Geometry check sheet. Reference: the model listing, model coordinates, mm. A direction names the side the tool comes from. Coordinates: 2 decimals unless noted, no trailing zeros. Write each loop counter-clockwise with the first axis right and the second up, starting at its lowest first coordinate (ties: lowest second). Pieces come first, ordered by that corner, then holes. Notation, with made-up numbers: M 35,66.5 L 92,66.5 A17 ccw 92,89.5 Z; hole C 66.25,75.25 d1. An arc over 180 degrees is marked long. Write item = value, one per line. Start each with the question number.
```python
from build123d import *

# Parameters (mm, degrees)
BOX017_W      = 3
BOX017_H      = 3
BOX017_DEPTH  = 3
BOX018_W      = 3
BOX018_H      = 3
BOX018_DEPTH  = 3
BOX019_W      = 3
BOX019_H      = 3
BOX019_DEPTH  = 3
BOX016_W      = 3
BOX016_H      = 3
BOX016_DEPTH  = 3
BOX012_W      = 3.1
BOX012_H      = 6
BOX012_DEPTH  = 10
BOX013_W      = 3.1
BOX013_H      = 6
BOX013_DEPTH  = 10
BOX014_W      = 6
BOX014_H      = 3.1
BOX014_DEPTH  = 10
BOX015_W      = 6
BOX015_H      = 3.1
BOX015_DEPTH  = 10
BOX001_W      = 3.1
BOX001_H      = 6
BOX001_DEPTH  = 3
BOX002_W      = 6
BOX002_H      = 3.1
BOX002_DEPTH  = 3
BOX003_W      = 6
BOX003_H      = 3.1
BOX003_DEPTH  = 3
BOX_W         = 3.1
BOX_H         = 6
BOX_DEPTH     = 3
TUBE001_R     = 16.7
TUBE001_R_2   = 15.7
TUBE001_DEPTH = 10
BOX005_W      = 1
BOX005_H      = 16
BOX005_DEPTH  = 10
BOX006_W      = 1
BOX006_H      = 16
BOX006_DEPTH  = 10
BOX007_W      = 1
BOX007_H      = 16
BOX007_DEPTH  = 10
BOX008_W      = 16
BOX008_H      = 1
BOX008_DEPTH  = 10
BOX009_W      = 16
BOX009_H      = 1
BOX009_DEPTH  = 10
BOX010_W      = 16
BOX010_H      = 1
BOX010_DEPTH  = 10
BOX011_W      = 16
BOX011_H      = 1
BOX011_DEPTH  = 10
BOX004_W      = 1
BOX004_H      = 16
BOX004_DEPTH  = 10
TUBE_R        = 32.5
TUBE_R_2      = 15.7
TUBE_DEPTH    = 3


with BuildPart() as finlock002:
    # Box017 → Box017 (new body)
    with BuildSketch(Plane(origin=(-1.5, 21, -3), x_dir=(1, 0, 0), z_dir=(0, 0, 1))):
        with Locations((1.5, 1.5)):
            Rectangle(BOX017_W, BOX017_H)
    extrude(amount=BOX017_DEPTH)


with BuildPart() as finlock003:
    # Box018 → Box018 (new body)
    with BuildSketch(Plane(origin=(-1.5, -24, -3), x_dir=(1, 0, 0), z_dir=(0, 0, 1))):
        with Locations((1.5, 1.5)):
            Rectangle(BOX018_W, BOX018_H)
    extrude(amount=BOX018_DEPTH)


with BuildPart() as finlock004:
    # Box019 → Box019 (new body)
    with BuildSketch(Plane(origin=(-24, -1.5, -3), x_dir=(1, 0, 0), z_dir=(0, 0, 1))):
        with Locations((1.5, 1.5)):
            Rectangle(BOX019_W, BOX019_H)
    extrude(amount=BOX019_DEPTH)


with BuildPart() as finlocks:
    # Box016 → Box016 (new body)
    with BuildSketch(Plane(origin=(21, -1.5, -3), x_dir=(1, 0, 0), z_dir=(0, 0, 1))):
        with Locations((1.5, 1.5)):
            Rectangle(BOX016_W, BOX016_H)
    extrude(amount=BOX016_DEPTH)

    # Fusion005: union FinLock002, FinLock003, FinLock004
    add(finlock002.part)
    add(finlock003.part)
    add(finlock004.part)


with BuildPart() as fincut005:
    # Box012 → Box012 (new body)
    with BuildSketch(Plane(origin=(-1.55, -21, -10), x_dir=(1, 0, 0), z_dir=(0, 0, 1))):
        with Locations((1.55, 3)):
            Rectangle(BOX012_W, BOX012_H)
    extrude(amount=BOX012_DEPTH)


with BuildPart() as fincut006:
    # Box013 → Box013 (new body)
    with BuildSketch(Plane(origin=(-1.55, 15, -10), x_dir=(1, 0, 0), z_dir=(0, 0, 1))):
        with Locations((1.55, 3)):
            Rectangle(BOX013_W, BOX013_H)
    extrude(amount=BOX013_DEPTH)


with BuildPart() as fincut007:
    # Box014 → Box014 (new body)
    with BuildSketch(Plane(origin=(15, -1.55, -10), x_dir=(1, 0, 0), z_dir=(0, 0, 1))):
        with Locations((3, 1.55)):
            Rectangle(BOX014_W, BOX014_H)
    extrude(amount=BOX014_DEPTH)


with BuildPart() as innerfincutouts:
    # Box015 → Box015 (new body)
    with BuildSketch(Plane(origin=(-21, -1.55, -10), x_dir=(1, 0, 0), z_dir=(0, 0, 1))):
        with Locations((3, 1.55)):
            Rectangle(BOX015_W, BOX015_H)
    extrude(amount=BOX015_DEPTH)

    # Fusion002: union FinCut005, FinCut006, FinCut007
    add(fincut005.part)
    add(fincut006.part)
    add(fincut007.part)


with BuildPart() as fincut002:
    # Box001 → Box001 (new body)
    with BuildSketch(Plane(origin=(-1.55, 28, 0), x_dir=(1, 0, 0), z_dir=(0, 0, 1))):
        with Locations((1.55, 3)):
            Rectangle(BOX001_W, BOX001_H)
    extrude(amount=BOX001_DEPTH)


with BuildPart() as fincut003:
    # Box002 → Box002 (new body)
    with BuildSketch(Plane(origin=(28, -1.55, 0), x_dir=(1, 0, 0), z_dir=(0, 0, 1))):
        with Locations((3, 1.55)):
            Rectangle(BOX002_W, BOX002_H)
    extrude(amount=BOX002_DEPTH)


with BuildPart() as fincut004:
    # Box003 → Box003 (new body)
    with BuildSketch(Plane(origin=(-34, -1.55, 0), x_dir=(1, 0, 0), z_dir=(0, 0, 1))):
        with Locations((3, 1.55)):
            Rectangle(BOX003_W, BOX003_H)
    extrude(amount=BOX003_DEPTH)


with BuildPart() as fincutouts:
    # Box → Box (new body)
    with BuildSketch(Plane(origin=(-1.55, -34, 0), x_dir=(1, 0, 0), z_dir=(0, 0, 1))):
        with Locations((1.55, 3)):
            Rectangle(BOX_W, BOX_H)
    extrude(amount=BOX_DEPTH)

    # Fusion: union FinCut002, FinCut003, FinCut004
    add(fincut002.part)
    add(fincut003.part)
    add(fincut004.part)

    # Fusion003: union InnerFinCutouts
    add(innerfincutouts.part)


with BuildPart() as innertube:
    # Tube001 → Tube001 (new body)
    with BuildSketch(Plane.XY.offset(-10)):
        Circle(TUBE001_R)
        Circle(TUBE001_R_2, mode=Mode.SUBTRACT)
    extrude(amount=TUBE001_DEPTH)


with BuildPart() as alignment002:
    # Box005 → Box005 (new body)
    with BuildSketch(Plane(origin=(-2.7, 16, -10), x_dir=(1, 0, 0), z_dir=(0, 0, 1))):
        with Locations((0.5, 8)):
            Rectangle(BOX005_W, BOX005_H)
    extrude(amount=BOX005_DEPTH)


with BuildPart() as alignment003:
    # Box006 → Box006 (new body)
    with BuildSketch(Plane(origin=(-2.7, -32, -10), x_dir=(1, 0, 0), z_dir=(0, 0, 1))):
        with Locations((0.5, 8)):
            Rectangle(BOX006_W, BOX006_H)
    extrude(amount=BOX006_DEPTH)


with BuildPart() as alignment004:
    # Box007 → Box007 (new body)
    with BuildSketch(Plane(origin=(1.7, -32, -10), x_dir=(1, 0, 0), z_dir=(0, 0, 1))):
        with Locations((0.5, 8)):
            Rectangle(BOX007_W, BOX007_H)
    extrude(amount=BOX007_DEPTH)


with BuildPart() as alignment005:
    # Box008 → Box008 (new body)
    with BuildSketch(Plane(origin=(16, 1.7, -10), x_dir=(1, 0, 0), z_dir=(0, 0, 1))):
        with Locations((8, 0.5)):
            Rectangle(BOX008_W, BOX008_H)
    extrude(amount=BOX008_DEPTH)


with BuildPart() as alignment006:
    # Box009 → Box009 (new body)
    with BuildSketch(Plane(origin=(16, -2.7, -10), x_dir=(1, 0, 0), z_dir=(0, 0, 1))):
        with Locations((8, 0.5)):
            Rectangle(BOX009_W, BOX009_H)
    extrude(amount=BOX009_DEPTH)


with BuildPart() as alignment007:
    # Box010 → Box010 (new body)
    with BuildSketch(Plane(origin=(-32, 1.7, -10), x_dir=(1, 0, 0), z_dir=(0, 0, 1))):
        with Locations((8, 0.5)):
            Rectangle(BOX010_W, BOX010_H)
    extrude(amount=BOX010_DEPTH)


with BuildPart() as alignment008:
    # Box011 → Box011 (new body)
    with BuildSketch(Plane(origin=(-32, -2.7, -10), x_dir=(1, 0, 0), z_dir=(0, 0, 1))):
        with Locations((8, 0.5)):
            Rectangle(BOX011_W, BOX011_H)
    extrude(amount=BOX011_DEPTH)


with BuildPart() as alignmenttabs:
    # Box004 → Box004 (new body)
    with BuildSketch(Plane(origin=(1.7, 16, -10), x_dir=(1, 0, 0), z_dir=(0, 0, 1))):
        with Locations((0.5, 8)):
            Rectangle(BOX004_W, BOX004_H)
    extrude(amount=BOX004_DEPTH)

    # Fusion001: union Alignment002, Alignment003, Alignment004, Alignment005, Alignment006, Alignment007, Alignment008
    add(alignment002.part)
    add(alignment003.part)
    add(alignment004.part)
    add(alignment005.part)
    add(alignment006.part)
    add(alignment007.part)
    add(alignment008.part)


with BuildPart() as obj1:
    # Tube → Tube (new body)
    with BuildSketch(Plane.XY):
        Circle(TUBE_R)
        Circle(TUBE_R_2, mode=Mode.SUBTRACT)
    extrude(amount=TUBE_DEPTH)

    # Fusion004: union InnerTube, AlignmentTabs
    add(innertube.part)
    add(alignmenttabs.part)

    # Cut: cut FinCutouts
    add(fincutouts.part, mode=Mode.SUBTRACT)

    # Connect: union FinLocks
    add(finlocks.part)


solid = obj1.part
```
Q1. Scan lines: L1, parallel to Y at x = 0, z = -1; L2, parallel to X at y = -25, z = -7. Record each from-to range of solid material in increasing order.
Q2. Cross-section at D-D on y = 12.5. Enter the section's corners in (x, z).
Q3. Set-up check for faces 4 (the face through (-23, 0, -3)), 5 (the face through (24, -1.7, -5)), 6 (the face through (-24, 2.7, -5)), 7 (the face through (2.7, -24, -5)), 8 (the face through (-30, -1.55, 1)): record each of +Z, -Z, +X, -X, +Y, -Y from which the full face is reachable in a straight line by a thin tool's end or side.
Q4. Gauge pin test, flat ends, axial feed: pin 1 (0.5 mm diameter, centred on x = 2.5, z = -3, fed in from -Y); pin 2 (3 mm diameter, centred on x = 20.5, z = -2.5, fed in from -Y); pin 3 (0.9 mm diameter, centred on x = 0, z = -1.5, fed in from +Y). Record the tip position at first contact, or that the pin passes through.
Q5. Draft check along X on faces 1 (the face through (0, -24, -2)), 2 (the face through (2.7, 24, -5)), 3 (the face through (30, 1.55, 1)). Enter one of: pulls with the +X half, pulls with the -X half, needs draft (parallel to the pull), parting line crosses it, or undercut.
Q6. Cross-section at C-C on z = -0.75. Count the separate pieces of the cut face and the enclosed holes in it, and give its area (3 significant figures).
Q7. Cross-section at A-A on x = 0. Enter the section's corners in (y, z).
Values found:
q1.L1 = -24 to -21, 21 to 24
q1.L2 = -2.7 to -1.7, 1.7 to 2.7
q2.outline = M -30,0 L -11.07,0 L -11.07,-10 L -9.5,-10 L -9.5,3 L -30,3 Z; M 9.5,-10 L 11.07,-10 L 11.07,0 L 30,0 L 30,3 L 9.5,3 Z
q3.face_4 = -Z, +X, -X
q3.face_5 = -Z, +X
q3.face_6 = -Z, -X, +Y
q3.face_7 = -Z, +X, -Y
q3.face_8 = +Z, -Z, -X
q4.pin_1 = -32
q4.pin_2 = -2.7
q4.pin_3 = 24
q5.face_1 = undercut
q5.face_2 = pulls with the +X half
q5.face_3 = needs draft
q6.separate_pieces = 8
q6.enclosed_holes = 0
q6.area = 249 mm²
q7.outline = M -28,0 L -24,0 L -24,-3 L -21,-3 L -21,0 L -15.7,0 L -15.7,3 L -28,3 Z; M 15.7,0 L 21,0 L 21,-3 L 24,-3 L 24,0 L 28,0 L 28,3 L 15.7,3 Z
